Part model, mm, in its own coordinate system. Face numbers are marked on the shaded views. A direction names the side the tool comes from. Coordinates: 2 decimals unless noted, no trailing zeros. Write each loop counter-clockwise with the first axis right and the second up, starting at its lowest first coordinate (ties: lowest second). Pieces come first, ordered by that corner, then holes. Notation, with made-up numbers: (-11.75, -34.5) -> (-7.75, -34.5) arc R28 cw to (-7.75, -15.5) -> close; hole circle Ø6 at (13, -23). An arc over 180 degrees is marked (long way). Write item = value, one per line. Start each with the question number.
Q1. Tool access for the marked faces 1, 2 and 3: list every direction of +Z, -Z, +X, -X, +Y, -Y with a clear straight run to the whole face (end or side of a thin tool).
Q2. Band-saw the part on B-B, the plane y = 199. List the corners of the cut face in (x, z) (3 decimals).
Q3. Band-saw the part on A-A, the plane x = 25.5. List the corners of the cut face in (y, z) (3 decimals).
Q4. Pull direction Y, two halves, no side cores. Call the marked faces 4, 5 and 6: released by +Y, released by -Y, zero draft, split by the parting line, or undercut.
Q5. Pin check, flat tips, straight feed: P1, Ø7.5, axis at x = 40.5, y = 281, coming from the -Z side; P2, Ø12.5, axis at x = -102, z = -523, coming from the -Y side (3 decimals); P3, Ø6, axis at x = -271, z = -317, coming from the -Y side (3 decimals). Stop position of each tip, or through.
Q6. Band-saw the part on C-C, the plane z = -96. List the corners of the cut face in (x, y) (3 decimals), plus the area to 3 significant figures.
Q7. Band-saw the part on D-D, the plane y = -683.5. List the corners of the cut face in (x, z) (3 decimals), plus the area to 3 significant figures.
Q8. Probe line 1 (Y direction, x = -464, z = -485.5) (3 decimals); line 2 (X direction, y = -68, z = -703.5) (3 decimals); line 3 (Z direction, x = 105, y = 177) (3 decimals). List the from-to ranges inside material, lowest first.
from build123d import *

# Parameters (mm, degrees)
F0_W      = 1219.2
F0_H      = 609.6
F1_DEPTH  = 15.875
F3_DEPTH  = 736.6
F4_W      = 1187.45
F4_H      = 15.875
F5_DEPTH  = 25.4
F6_W      = 898.525
F6_H      = 127
F7_DEPTH  = 25.4
F9_DEPTH  = 609.6
F10_W     = 15.875
F10_H     = 736.6
F11_DEPTH = 288.925
F12_W     = 203.2
F12_H     = 15.875
F13_DEPTH = 1187.45
F14_W     = 203.2
F14_H     = 15.875
F15_DEPTH = 984.25


with BuildPart() as f1:
    # F0 (on Top) → F1 (new body)
    with BuildSketch(Plane.XY):
        Rectangle(F0_W, F0_H)
    extrude(amount=F1_DEPTH)

    # F2 (on face) → F3 (join)
    with BuildSketch(Plane(origin=(0, 0, 0), x_dir=(1, 0, 0), z_dir=(0, 0, -1))):
        Polygon((593.725, -288.925), (-593.725, -288.925), (-593.725, 304.8), (-609.6, 304.8), (-609.6, -304.8), (609.6, -304.8), (609.6, 304.8), (593.725, 304.8), align=None)
    extrude(amount=F3_DEPTH)

    # F4 (on face) → F5 (join)
    with BuildSketch(Plane.XZ.offset(-288.925)):
        with Locations((0, -134.9375)):
            Rectangle(F4_W, F4_H)
    extrude(amount=F5_DEPTH)

    # F6 (on face) → F7 (cut)
    with BuildSketch(Plane.XZ.offset(-288.925)):
        with Locations((144.4625, -63.5)):
            Rectangle(F6_W, F6_H)
    extrude(amount=-F7_DEPTH, mode=Mode.SUBTRACT)

    # F8 (on face) → F9 (join)
    with BuildSketch(Plane.XZ.offset(304.8)):
        Polygon((-304.8, 0), (-304.8, 15.875), (-609.6, 15.875), (-609.6, -736.6), (-593.725, -736.6), (-593.725, 0), align=None)
    extrude(amount=F9_DEPTH)

    # F10 (on face) → F11 (join)
    with BuildSketch(Plane.YZ.offset(-593.725)):
        with Locations((-906.4625, -368.3)):
            Rectangle(F10_W, F10_H)
    extrude(amount=F11_DEPTH)

    # F12 (on face) → F13 (join)
    with BuildSketch(Plane(origin=(0, -898.525, 0), x_dir=(-1, 0, 0), z_dir=(0, 1, 0))):
        with Locations((492.125, -525.4625)):
            Rectangle(F12_W, F12_H)
    extrude(amount=F13_DEPTH)

    # F14 (on face) → F15 (join)
    with BuildSketch(Plane.YZ.offset(-390.525)):
        with Locations((187.325, -525.4625)):
            Rectangle(F14_W, F14_H)
    extrude(amount=F15_DEPTH)


solid = f1.part
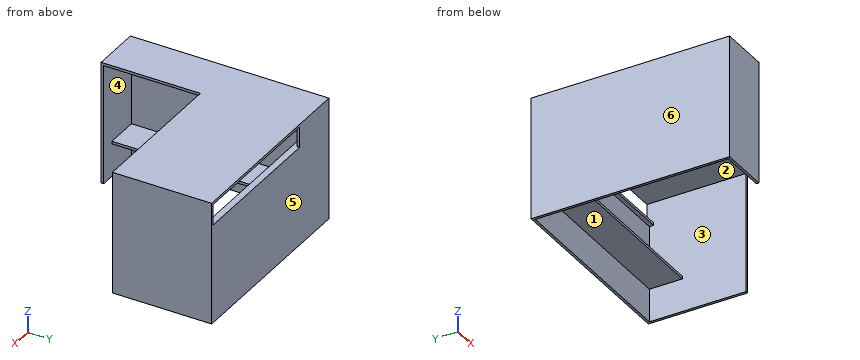
Ans:
q1.face_1 = -Z
q1.face_2 = none
q1.face_3 = -Y
q2.outline = (-609.6, -736.6) -> (-593.725, -736.6) -> (-593.725, -533.4) -> (593.725, -533.4) -> (593.725, -736.6) -> (609.6, -736.6) -> (609.6, 15.875) -> (-609.6, 15.875) -> close; hole (-593.725, -517.525) -> (593.725, -517.525) -> (593.725, 0) -> (-593.725, 0) -> close
q3.outline = (-304.8, 0) -> (304.8, 0) -> (304.8, 15.875) -> (-304.8, 15.875) -> close; (85.725, -533.4) -> (288.925, -533.4) -> (288.925, -736.6) -> (304.8, -736.6) -> (304.8, -127) -> (263.525, -127) -> (263.525, -142.875) -> (288.925, -142.875) -> (288.925, -517.525) -> (85.725, -517.525) -> close
q4.face_4 = undercut
q4.face_5 = released by +Y
q4.face_6 = zero draft
q5.P1 = -533.4
q5.P2 = 85.725
q5.P3 = 288.925
q6.outline = (-609.6, -914.4) -> (-304.8, -914.4) -> (-304.8, -898.525) -> (-593.725, -898.525) -> (-593.725, 288.925) -> (-304.8, 288.925) -> (-304.8, 304.8) -> (-609.6, 304.8) -> close; (593.725, -304.8) -> (609.6, -304.8) -> (609.6, 304.8) -> (593.725, 304.8) -> close
q6.area = 38,200 mm2
q7.outline = (-609.6, -736.6) -> (-593.725, -736.6) -> (-593.725, -533.4) -> (-390.525, -533.4) -> (-390.525, -517.525) -> (-593.725, -517.525) -> (-593.725, 0) -> (-304.8, 0) -> (-304.8, 15.875) -> (-609.6, 15.875) -> close
q7.area = 19,800 mm2
q8.line_1 = -914.4 to -898.525, 288.925 to 304.8
q8.line_2 = -609.6 to -593.725, 593.725 to 609.6
q8.line_3 = -533.4 to -517.525, 0 to 15.875
